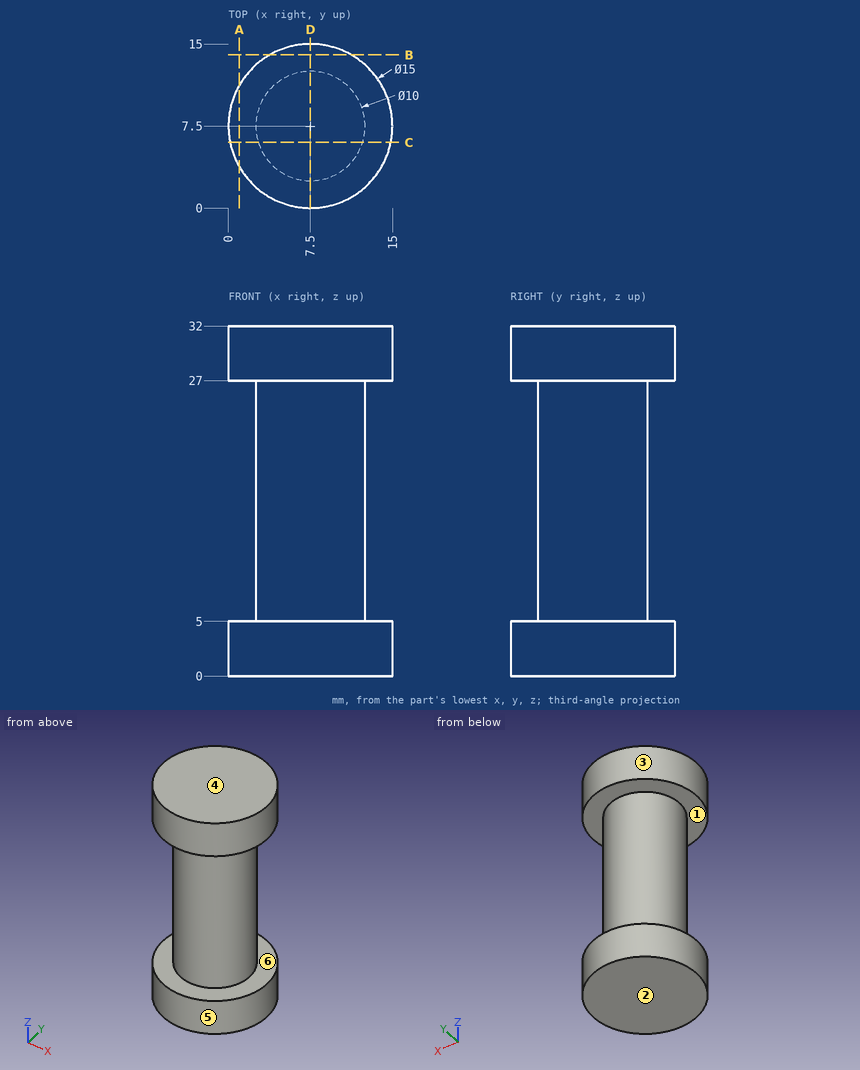
Geometry check sheet. Reference: drawing and pictorial views, mm from the part's lowest x, y, z. A direction names the side the tool comes from. Round coordinates to 2 decimals unless told otherwise and drop trailing zeros. Order: outer loops, then holes, each group sorted by start corner. A loop starts at its lowest first (then second) coordinate and runs counter-clockwise, first axis right, second up. Notation, with made-up numbers: (-36.75, -17) -> (-1.75, -17) arc R27 ccw to (-1.75, 4) -> close; hole circle Ø11 at (57.25, 85). An arc over 180 degrees is marked (long way). One line per item, written item: value. Start each with the question number.
Q1. Cross-section at C-C (y = 6). Record the boundary of the cut face in (x, z).
Q2. Set-up check for the marked faces 5 and 6: record each of +Z, -Z, +X, -X, +Y, -Y from which the full face is reachable in a straight line by a thin tool's end or side.
Q3. Gauge pin test, flat ends, axial feed: pin 1 Ø8 at (x, z) = (3.5, 11.5) entering from +Y; pin 2 Ø1 at (x, y) = (4, 4.5) entering from -Z. Record the tip position at first contact, or that the pin passes through.
Q4. Mould release check, pull along Z, two halves, no side actions. Record for the marked faces 1, 2, 3 and 4: pulls with the +Z half, pulls with the -Z half, needs draft (parallel to the pull), parting line crosses it, or undercut.
Q5. Cross-section at A-A (x = 1). Record the boundary of the cut face in (y, z).
Q6. Cross-section at D-D (x = 7.5). Record the boundary of the cut face in (y, z).
Q7. Thickness scan on line 1 (Z direction, x = 1.5, y = 10); line 2 (Y direction, x = 7.5, z = 11); line 3 (Y direction, x = 10.25, z = 25.5). Record the ranges inside material, lowest first.
Completed:
1. outline: (0.15, 0) -> (14.85, 0) -> (14.85, 5) -> (12.27, 5) -> (12.27, 27) -> (14.85, 27) -> (14.85, 32) -> (0.15, 32) -> (0.15, 27) -> (2.73, 27) -> (2.73, 5) -> (0.15, 5) -> close
2. face 5: +Z, -Z
2. face 6: none
3. pin 1: stops at y = 12.5
3. pin 2: stops at z = 0
4. face 1: undercut
4. face 2: pulls with the -Z half
4. face 3: needs draft
4. face 4: pulls with the +Z half
5. outline: (3.76, 0) -> (11.24, 0) -> (11.24, 5) -> (3.76, 5) -> close; (3.76, 27) -> (11.24, 27) -> (11.24, 32) -> (3.76, 32) -> close
6. outline: (0, 0) -> (15, 0) -> (15, 5) -> (12.5, 5) -> (12.5, 27) -> (15, 27) -> (15, 32) -> (0, 32) -> (0, 27) -> (2.5, 27) -> (2.5, 5) -> (0, 5) -> close
7. line 1: z = 0 to 5, 27 to 32
7. line 2: y = 2.5 to 12.5
7. line 3: y = 3.32 to 11.68
